Input: part model. Units: mm. Frame: model coordinates. Face numbers are marked on the shaded views. Give positions to 0.01 mm unless a question says otherwise; leave off trailing zeros. Write each loop counter-clockwise with the first axis right and the second up, starting at its lowest first coordinate (ties: lowest second). Pieces come first, ordered by that corner, then holes. Notation, with made-up numbers: (-30.75, 83.25) - (12.25, 83.25) arc R17 ccw to (12.25, 114.25) - close; hole circle Ø5 at (44, 73.5). An arc over 180 degrees is marked (long way). Answer as CSV lines item,"result".
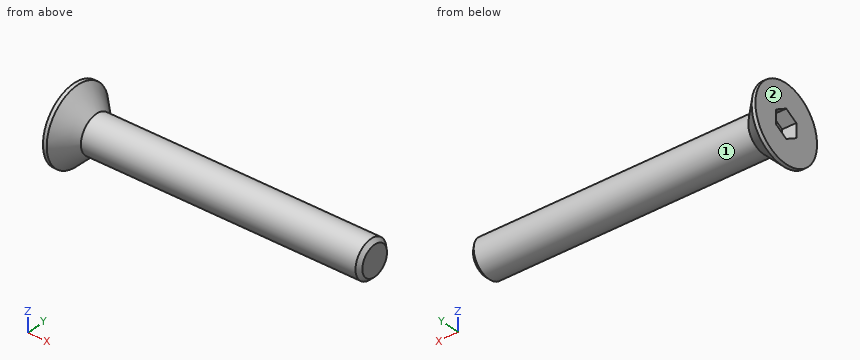
```python
from build123d import *

# Parameters (mm, degrees)
CHAMFER1_SIZE      = 0.2
CUT_EXTRUDE1_DEPTH = 0.75


with BuildPart() as part:
    # Sketch1 → Revolve1 (revolve)
    with BuildSketch(Plane.XY):
        Polygon((0, 1), (-1, 2), (-1.2, 2), (-1.2, 0), (14.8, 0), (14.8, 1), align=None)
    revolve(axis=Axis((-1.2, 0, 0), (1, 0, 0)))

    # Chamfer1
    chamfer1_edges = [part.edges().sort_by_distance(p)[0] for p in [
        (14.8, -1, 0),
    ]]
    chamfer(chamfer1_edges, length=CHAMFER1_SIZE)

    # Sketch2 → Cut-Extrude1 (cut)
    with BuildSketch(Plane.ZY.offset(1.2)):
        Polygon((-0.75055535, 0), (-0.375277675, -0.65), (0.375277675, -0.65), (0.75055535, 0), (0.375277675, 0.65), (-0.375277675, 0.65), align=None)
    extrude(amount=-CUT_EXTRUDE1_DEPTH, mode=Mode.SUBTRACT)


solid = part.part
```
Item 1: Mould query, pull axis Y, two halves, no side actions, for the marked faces 1 and 2. Classes: +Y half, -Y half, draft (parallel to the pull), parting line (faces both ways), or undercut.
The answers:
face 1,"parting line"
face 2,"draft"
Item 2: Cut plane B-B on x = 4.5. Return the cut outline in (y, z), plus the area to 3 significant figures.
The answers:
outline,"circle Ø2 at (0, 0)"
area,"3.14 mm²"
Item 3: Contact query for flat-ended pins moving along their axis: pin 1 (1.4 mm diameter, centred on y = 0, z = 0, fed in from -X); pin 2 (1.5 mm diameter, centred on x = 10, y = -1, fed in from -Z); pin 3 (1.5 mm diameter, centred on x = 1, y = 1.5, fed in from +Z). Output: stop coordinate, or through.
The answers:
pin 1,"x = -1.2"
pin 2,"z = -0.97"
pin 3,"z = 0.66"
Item 4: Ray query, line 1 (X direction, y = -0.3, z = -0.3); line 2 (Z direction, x = 4.25, y = 0.6); line 3 (X direction, y = 1.45, z = -0.7). Return the intervals inside material, ascending. Write a range as from..to.
The answers:
line 1,"-0.45..14.8"
line 2,"-0.8..0.8"
line 3,"-1.2..-0.61"
Item 5: Cut plane A-A on z = 0. Return the cut outline in (x, y), plus the area to 3 significant figures.
The answers:
outline,"(-1.2, -2) - (-1, -2) - (0, -1) - (14.6, -1) - (14.8, -0.8) - (14.8, 0.8) - (14.6, 1) - (0, 1) - (-1, 2) - (-1.2, 2) - (-1.2, 0.65) - (-0.45, 0.65) - (-0.45, -0.65) - (-1.2, -0.65) - close"
area,"32.4 mm²"
